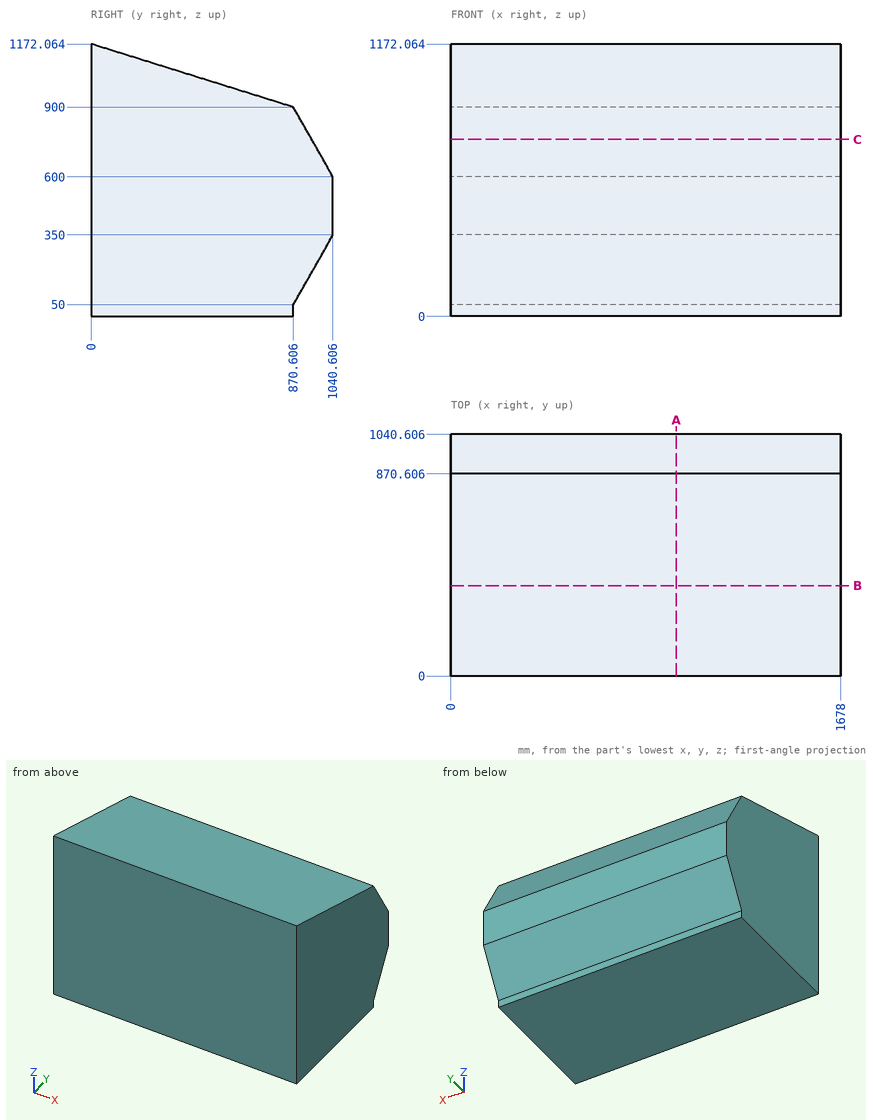
For this review, use the dimensioned drawing (mm, ordinates from the lowest corner) and the shaded views. Coordinates: 2 decimals unless noted, no trailing zeros. Write each loop counter-clockwise with the first axis right and the second up, starting at its lowest first coordinate (ties: lowest second). Pieces come first, ordered by that corner, then holes. Notation, with made-up numbers: (82.5, 23) - (111.5, 23) arc R22 ccw to (111.5, 39) - close; hole circle Ø3 at (20, -31.75). An arc over 180 degrees is marked (long way). One line per item, written item: value.
1) To check wall thickness, follow probe 1 along Y at (x, z) = (164, 684) (1 decimal); probe 2 along Z at (x, y) = (301, 772) (1 decimal); probe 3 along Z at (x, y) = (999, 127). State the ranges of each line that lie inside material, in increasing order.
Answer sheet:
probe 1: y = 0 to 993
probe 2: z = 0 to 930.8
probe 3: z = 0 to 1132.38
2) Add section B-B (y = 389.5). State the section outline as (x, z) points (1 decimal), plus the area to 3 significant figures.
Answer sheet:
outline: (0, 0) - (1678, 0) - (1678, 1050.3) - (0, 1050.3) - close
area: 1,760,000 mm2
3) Add section C-C (z = 762). State the section outline as (x, y) points.
Answer sheet:
outline: (0, 0) - (1678, 0) - (1678, 948.81) - (0, 948.81) - close
4) Add section A-A (x = 970.5). State the section outline as (y, z) points (1 decimal).
Answer sheet:
outline: (0, 0) - (870.6, 0) - (870.6, 50) - (1040.6, 350) - (1040.6, 600) - (870.6, 900) - (0, 1172.1) - close
5) Insertion check: pin 1 (3 mm diameter, centred on x = 927.5, z = 223, fed in from +Y); pin 2 (15 mm diameter, centred on x = 1209.5, z = 34.5, fed in from +Y); pin 3 (12 mm diameter, centred on x = 687, z = 882.5, fed in from +Y); pin 4 (4 mm diameter, centred on x = 1078, y = 119, fed in from -Z). Each pin has a flat end and moves straight along its axis. Give the tip position at first contact, or say it passes through.
Answer sheet:
pin 1: stops at y = 969.49
pin 2: stops at y = 870.61
pin 3: stops at y = 883.92
pin 4: stops at z = 0
